```python
from build123d import *

# Parameters (mm, degrees)
F0_W      = 110
F0_H      = 73
F1_DEPTH  = 13.8
F2_W      = 84
F2_H      = 54
F3_DEPTH  = 10.8
F4_W      = 10
F4_H      = 73
F5_DEPTH  = 8
F6_R      = 1.75
F7_DEPTH  = 25
F8_R      = 3
F9_DEPTH  = 5
F10_W     = 64.3
F10_H     = 14.4
F10_W_2   = 24
F10_W_3   = 14
F10_H_2   = 10
F11_DEPTH = 25
F12_W     = 11.6
F12_H     = 9.5
F13_DEPTH = 25
F15_START = -27.4
F15_DEPTH = 10


# Not quite as in the source:
# - a pattern or mirror of a feature is missing from the dataset's text; its kind, count and spacing are read off the source's solid


with BuildPart() as f1:
    # F0 (on Top) → F1 (new body)
    with BuildSketch(Plane.XY):
        with Locations((55, 36.5)):
            Rectangle(F0_W, F0_H)
    extrude(amount=F1_DEPTH)

    # F2 (on face) → F3 (cut)
    with BuildSketch(Plane(origin=(0, 0, 0), x_dir=(1, 0, 0), z_dir=(0, 0, -1))):
        with Locations((58, -37)):
            Rectangle(F2_W, F2_H)
    extrude(amount=-F3_DEPTH, mode=Mode.SUBTRACT)

    # F4 (on face) → F5 (join)
    with BuildSketch(Plane(origin=(0, 0, 0), x_dir=(1, 0, 0), z_dir=(0, 0, -1))):
        with Locations((105, -36.5)):
            Rectangle(F4_W, F4_H)
    extrude(amount=F5_DEPTH)

    # F6 (on face) → F7 (cut)
    with BuildSketch(Plane.XY.offset(13.8)):
        with Locations((5.85, 5)):
            Circle(F6_R)
        with Locations((94.15, 5)):
            Circle(F6_R)
        with Locations((94.15, 68.5)):
            Circle(F6_R)
        with Locations((5.85, 68.5)):
            Circle(F6_R)
    extrude(amount=-F7_DEPTH, mode=Mode.SUBTRACT)

    # F8 (on face) → F9 (cut)
    with BuildSketch(Plane.XY.offset(13.8)):
        with Locations((5.85, 68.5)):
            Circle(F8_R)
        with Locations((5.85, 5)):
            Circle(F8_R)
        with Locations((94.15, 5)):
            Circle(F8_R)
        with Locations((94.15, 68.5)):
            Circle(F8_R)
    extrude(amount=-F9_DEPTH, mode=Mode.SUBTRACT)

    # F10 (on face) → F11 (cut)
    with BuildSketch(Plane.XY.offset(13.8)):
        with Locations((58.15, 32.6)):
            Rectangle(F10_W, F10_H)
        with Locations((80.48, 55.3)):
            Rectangle(F10_W_2, F10_H)
        with Locations((32.8, 52.7)):
            Rectangle(F10_W_3, F10_H_2)
    extrude(amount=-F11_DEPTH, mode=Mode.SUBTRACT)

    # F12 (on face) → F13 (cut)
    with BuildSketch(Plane.YZ.offset(110)):
        with Locations((43.2, -3.25)):
            Rectangle(F12_W, F12_H)
    extrude(amount=-F13_DEPTH, mode=Mode.SUBTRACT)

    # F14 (on face) → F15 (join)
    with BuildSketch(Plane.XZ.offset(F15_START)):
        Polygon((94, -8), (97.5, -8), (97.5, 2), (100, 2), (100, 4.5), (100, 13.8), (96, 13.8), (96, 4.5), (94, -1.75), align=None)
    f15 = extrude(amount=-F15_DEPTH)

    # F15_copies: F15 across plane
    add(f15.mirror(Plane.ZX.offset(43.2)))


solid = f1.part
```
Source: CAD feature listing. Evaluate the final solid. Frame: model axes, mm. A direction names the side the tool comes from. Give positions to 0.01 mm unless a question says otherwise; leave off trailing zeros. Write each loop counter-clockwise with the first axis right and the second up, starting at its lowest first coordinate (ties: lowest second). Pieces come first, ordered by that corner, then holes.
1. Section query B-B (y = 68.5). Return the cut outline in (x, z).
2. Section query A-A (x = 28). Return the cut outline in (y, z), then the cut area to 3 significant figures.
3. Section query D-D (x = 5.85). Return the cut outline in (y, z).
4. Material intervals for line 1 along Y through (x, z) = (73, 11.75); line 2 along Y through (x, z) = (94.15, 11.2); line 3 along X through (y, z) = (68.5, 4), sorted ascending.
5. Access query for faces 5 (the face through (16, 37, 5)), 6 (the face through (90.3, 32, 12)), 7 (the face through (105, 43, 1.5)), 8 (the face through (8, 69, 8.8)). Directions: +Z, -Z, +X, -X, +Y, -Y. A direction counts if a zero-diameter tool reaches every point of the face in a straight line with its end or side. Return the directions, or none.
6. Section query C-C (z = -3.25). Return the cut outline in (x, y).
7. First-contact query: pin 1 (0.8 mm diameter, centred on x = 99.5, y = 35, fed in from -Z); pin 2 (2 mm diameter, centred on x = 15.5, y = 54, fed in from -Z). Flat tips, straight axial feed; report the tip coordinate or a pass-through.
8. Pull-direction query (Y, two-part tool) for faces 1 (the face through (105, 18, -8)), 2 (the face through (57, 43, 10.8)), 3 (the face through (54, 73, 5)), 4 (the face through (91.769, 3.175, 11.335)); classes: +Y half, -Y half, draft (parallel to the pull), parting line (faces both ways), or undercut.
Output values:
1. outline: (0, 0) - (4.1, 0) - (4.1, 8.8) - (2.85, 8.8) - (2.85, 13.8) - (0, 13.8) - close; (7.6, 0) - (92.4, 0) - (92.4, 8.8) - (91.15, 8.8) - (91.15, 13.8) - (8.85, 13.8) - (8.85, 8.8) - (7.6, 8.8) - close; (95.9, 0) - (100, 0) - (100, -8) - (110, -8) - (110, 13.8) - (97.15, 13.8) - (97.15, 8.8) - (95.9, 8.8) - close
2. outline: (0, 0) - (10, 0) - (10, 10.8) - (25.4, 10.8) - (25.4, 13.8) - (0, 13.8) - close; (39.8, 10.8) - (47.7, 10.8) - (47.7, 13.8) - (39.8, 13.8) - close; (57.7, 10.8) - (64, 10.8) - (64, 0) - (73, 0) - (73, 13.8) - (57.7, 13.8) - close
2. area: 351 mm2
3. outline: (0, 0) - (3.25, 0) - (3.25, 8.8) - (2, 8.8) - (2, 13.8) - (0, 13.8) - close; (6.75, 0) - (66.75, 0) - (66.75, 8.8) - (65.5, 8.8) - (65.5, 13.8) - (8, 13.8) - (8, 8.8) - (6.75, 8.8) - close; (70.25, 0) - (73, 0) - (73, 13.8) - (71.5, 13.8) - (71.5, 8.8) - (70.25, 8.8) - close
4. line 1: y = 0 to 25.4, 39.8 to 48.1, 62.5 to 73
4. line 2: y = 0 to 2, 8 to 65.5, 71.5 to 73
4. line 3: x = 0 to 4.1, 7.6 to 92.4, 95.9 to 110
5. face 5: -Z
5. face 6: +Z, -Z
5. face 7: -Z, +X
5. face 8: +Z
6. outline: (94, 27.4) - (97.5, 27.4) - (97.5, 37.4) - (94, 37.4) - close; (94, 49) - (97.5, 49) - (97.5, 59) - (94, 59) - close; (100, 0) - (110, 0) - (110, 37.4) - (100, 37.4) - close; (100, 49) - (110, 49) - (110, 73) - (100, 73) - close
7. pin 1: stops at z = 2
7. pin 2: stops at z = 0
8. face 1: draft
8. face 2: undercut
8. face 3: +Y half
8. face 4: undercut
